Can you work these out from the model? Positions are in its coordinate system, mm. A direction names the side the tool comes from. Coordinates: 2 decimals unless noted, no trailing zeros. Order: outer loops, then holes, each group sorted by start corner. A loop starts at its lowest first (then second) coordinate and runs counter-clockwise, first axis right, second up. Notation, with made-up numbers: (-3.75, 1.25) -> (47.25, 1.25) arc R8 cw to (47.25, 12.25) -> close; hole circle Ø4 at (15.5, 23.25). An arc over 180 degrees is marked (long way). Answer in a Markdown table with one row per item.
```python
from build123d import *

# Parameters (mm, degrees)
F1_DEPTH = 40
F0_R     = 2
F2_DEPTH = 10


with BuildPart() as f1:
    # F0 (on Top) → F1 (new body)
    with BuildSketch(Plane.XY):
        with BuildLine():
            Line((-21.3541565041, -24.5), (0, -24.5))
            ThreePointArc((0, -24.5), (-23.6272833171, -6.4808551176), (-12.5, 21.0713075057))
            Line((-12.5, 21.0713075057), (-17.433109084, 27.4287569471))
            ThreePointArc((-17.433109084, 27.4287569471), (-32.4077451, 2.4470507823), (-21.3541565041, -24.5))
        make_face()
        with BuildLine():
            ThreePointArc((12.5, 21.0713075057), (21.289668856, 12.124355653), (24.5, 0))
            ThreePointArc((24.5, 0), (17.3241161391, -17.3241161391), (0, -24.5))
            Line((0, -24.5), (21.3541565041, -24.5))
            ThreePointArc((21.3541565041, -24.5), (29.582596965, -13.4580814684), (32.5, 0))
            ThreePointArc((32.5, 0), (28.4853124016, 15.6472674095), (17.433109084, 27.4287569471))
            Line((17.433109084, 27.4287569471), (12.5, 21.0713075057))
        make_face()
        with BuildLine():
            Line((21.3541565041, -24.5), (0, -24.5))
            Line((0, -24.5), (0, -32.5))
            ThreePointArc((0, -32.5), (11.401754251, -30.4343555871), (21.3541565041, -24.5))
        make_face()
        with BuildLine():
            Line((0, -32.5), (0, -24.5))
            Line((0, -24.5), (-21.3541565041, -24.5))
            ThreePointArc((-21.3541565041, -24.5), (-11.401754251, -30.4343555871), (0, -32.5))
        make_face()
    extrude(amount=-F1_DEPTH)

    # F0 (on Top) → F2 (join)
    with BuildSketch(Plane.XY):
        with BuildLine():
            Line((0, -54.5), (0, -32.5))
            ThreePointArc((0, -32.5), (-11.401754251, -30.4343555871), (-21.3541565041, -24.5))
            Line((-21.3541565041, -24.5), (-60, -24.5))
            Line((-60, -24.5), (-60, -54.5))
            Line((-60, -54.5), (0, -54.5))
        make_face()
        with Locations((-50.0000007451, -42.5000099838)):
            Circle(F0_R, mode=Mode.SUBTRACT)
        with BuildLine():
            ThreePointArc((21.3541565041, -24.5), (11.401754251, -30.4343555871), (0, -32.5))
            Line((0, -32.5), (0, -54.5))
            Line((0, -54.5), (60, -54.5))
            Line((60, -54.5), (60, -24.5))
            Line((60, -24.5), (21.3541565041, -24.5))
        make_face()
        with Locations((50.0000007451, -42.5000099838)):
            Circle(F0_R, mode=Mode.SUBTRACT)
    extrude(amount=-F2_DEPTH)


solid = f1.part
```
(1) Suppose I cut it at B-B (z = -22). Please give me the cut outline in (x, y).
Response values:
| item | result |
|---|---|
| outline | (-17.43, 27.43) arc R32.5 ccw (long way) to (17.43, 27.43) -> (12.5, 21.07) arc R24.5 cw (long way) to (-12.5, 21.07) -> close |
(2) Suppose I cut it at C-C (y = -23). Please give me the cut outline in (x, z).
Response values:
| item | result |
|---|---|
| outline | (-22.96, -40) -> (-8.44, -40) -> (-8.44, 0) -> (-22.96, 0) -> close; (8.44, -40) -> (22.96, -40) -> (22.96, 0) -> (8.44, 0) -> close |
(3) Will these pins go through, and if not, where does the flat tip stop? pin 1 Ø8 at (x, z) = (44, -2.5) entering from +Y; pin 2 Ø5 at (y, z) = (18.5, -30) entering from +X; pin 3 Ø9 at (x, y) = (-25.5, -45.5) entering from -Z.
Response values:
| item | result |
|---|---|
| pin 1 | y = -24.5 |
| pin 2 | x = 28.29 |
| pin 3 | z = -10 |
(4) I need wall thicknesses on line 1 (Y direction, x = -50, z = -2); line 2 (Z direction, x = 2, y = -32.5); line 3 (X direction, y = 24, z = -23.5). Which ranges of each line are inside material? Lowest first, please. Write a range as [from, to].
Response values:
| item | result |
|---|---|
| line 1 | [-54.5, -44.5], [-40.5, -24.5] |
| line 2 | [-10, 0] |
| line 3 | [-21.91, -14.77], [14.77, 21.91] |
(5) Suppose I cut it at D-D (y = -37). Please give me the cut outline in (x, z).
Response values:
| item | result |
|---|---|
| outline | (-60, -10) -> (60, -10) -> (60, 0) -> (-60, 0) -> close |
(6) We'd pull the mould along X, two halves only. Please class faces 5 (the flat face through (15, 24.29, -19.72)), 6 (the flat face through (60, -40, -5)), 7 (the flat face through (-1, -39, -10)): +X half, -X half, draft (parallel to the pull), parting line (faces both ways), or undercut.
Response values:
| item | result |
|---|---|
| face 5 | undercut |
| face 6 | +X half |
| face 7 | draft |
(7) Suppose I cut it at A-A (x = 50). Please give me the cut outline in (y, z).
Response values:
| item | result |
|---|---|
| outline | (-54.5, -10) -> (-44.5, -10) -> (-44.5, 0) -> (-54.5, 0) -> close; (-40.5, -10) -> (-24.5, -10) -> (-24.5, 0) -> (-40.5, 0) -> close |
(8) On a 3-axis mill with a long thin cutter (end or side, diameter ignored), from which of +Z, -Z, +X, -X, +Y, -Y can I reach the whole of each face in a straight line? I mean faces 1 (the flat face through (-14.932, 24.206, -19.72)), 2 (the flat face through (-40, -24.5, -5)), 3 (the flat face through (41, -24.5, -5)), 4 (the cylindrical face through (48.526, -41.148, -4.93)). Say none if no direction works.
Response values:
| item | result |
|---|---|
| face 1 | +Z, -Z, +Y |
| face 2 | +Z, -Z, -X |
| face 3 | +Z, -Z, +X |
| face 4 | +Z, -Z |
